```python
from build123d import *

# Parameters (mm, degrees)
F1_DEPTH       = 110
F0_W           = 30
F0_H           = 30
F2_DEPTH       = 3.36
F3_R           = 2
F5_D           = 8
F5_DEPTH       = 4
F7_D           = 4
F7_DEPTH       = 4
F7_CSINK_D     = 8
F7_CSINK_ANGLE = 90
F8_W           = 30
F8_H           = 13
F9_DEPTH       = 1


with BuildPart() as f1:
    # F0 (on Top) → F1 (new body)
    with BuildSketch(Plane.XY):
        Polygon((15, -18.36), (15, -15), (-15, -15), (-15, 15), (15, 15), (15, 18.36), (-18.36, 18.36), (-18.36, -18.36), align=None)
    extrude(amount=F1_DEPTH)

    # F0 (on Top) → F2 (join)
    with BuildSketch(Plane.XY):
        Rectangle(F0_W, F0_H)
    extrude(amount=F2_DEPTH)

    # F3
    f3_edges = [f1.edges().sort_by_distance(p)[0] for p in [
        (-18.36, -18.36, 55),
        (-18.36, 18.36, 55),
        (15, -18.36, 55),
        (15, 18.36, 55),
    ]]
    fillet(f3_edges, radius=F3_R)

    # F5
    with Locations(Plane.XZ.offset(18.36)):
        with Locations((0, 30), (0, 80)):
            Hole(F5_D / 2, depth=F5_DEPTH)

    # F7
    with Locations(Plane.XZ.offset(-15)):
        with Locations((0, 30), (0, 80)):
            CounterSinkHole(F7_D / 2, F7_CSINK_D / 2, depth=F7_DEPTH, counter_sink_angle=F7_CSINK_ANGLE)

    # F8 (on face) → F9 (cut)
    with BuildSketch(Plane(origin=(0, -15, 0), x_dir=(-1, 0, 0), z_dir=(0, 1, 0))):
        with Locations((0, 16.86)):
            Rectangle(F8_W, F8_H)
    extrude(amount=-F9_DEPTH, mode=Mode.SUBTRACT)


solid = f1.part
```
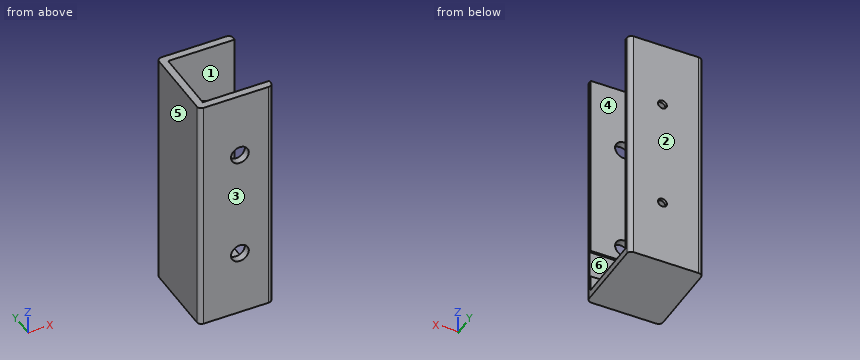
Read the model definition and answer for the solid it produces. Units are mm, in the model's axes. Face numbers are marked on the shaded views. A direction names the side the tool comes from. Coordinates: 2 decimals unless noted, no trailing zeros. Write each loop counter-clockwise with the first axis right and the second up, starting at its lowest first coordinate (ties: lowest second). Pieces come first, ordered by that corner, then holes. Notation, with made-up numbers: (85.25, -14) - (114.25, -14) arc R6 cw to (114.25, -10) - close; hole circle Ø11 at (-30.75, 79). An arc over 180 degrees is marked (long way). Answer as a JSON object with one key per item and string values. Group by question number.
1. The mould has two halves that part along Y. Classify the marked faces 1, 2 and 3: +Y half, -Y half, draft (parallel to the pull), parting line (faces both ways), or undercut.
2. A cutting plane is placed at D-D (z = 61.5). Determine the outline of the cut face in (x, y).
3. Each of these flat-tipped pins is pushed along its axis until it touches: P1, Ø8, axis at x = -2.5, y = -10.5, coming from the +Z side; P2, Ø4.5, axis at x = 0, z = 80, coming from the -Y side; P3, Ø12, axis at y = -7, z = 55.5, coming from the +X side. Where does it stop, or does it pass through?
4. A cutting plane is placed at C-C (y = -8). Determine the outline of the cut face in (x, z), plus the area to 3 significant figures.
5. Which of the six approach directions +Z, -Z, +X, -X, +Y, -Y give full straight-line access (tool end or side, diameter ignored) to the marked faces 4, 5 and 6?
6. A cutting plane is placed at B-B (x = 0). Give the number of separate pieces and of enclosed holes in the cut face, plus the area to 3 significant figures.
7. Consider L1, parallel to Z at x = 0, y = -16.95; L2, parallel to Y at x = -11, z = 34.5; L3, parallel to Z at x = 0, y = 17. Determine where each line is inside the solid, lowest interval first. Write a range as [from, to].
8. A cutting plane is placed at A-A (z = 30). Determine the outline of the cut face in (x, y), plus the area to 3 significant figures.
Worked out:
{
 "1": {"face 1": "undercut", "face 2": "+Y half", "face 3": "-Y half"},
 "2": {"outline": "(-18.36, -16.36) arc R2 ccw to (-16.36, -18.36) - (13, -18.36) arc R2 ccw to (15, -16.36) - (15, -15) - (-15, -15) - (-15, 15) - (15, 15) - (15, 16.36) arc R2 ccw to (13, 18.36) - (-16.36, 18.36) arc R2 ccw to (-18.36, 16.36) - close"},
 "3": {"P1": "stops at z = 3.36", "P2": "stops at y = 16.75", "P3": "stops at x = -15"},
 "4": {"outline": "(-18.36, 0) - (15, 0) - (15, 3.36) - (-15, 3.36) - (-15, 110) - (-18.36, 110) - close", "area": "470 mm²"},
 "5": {"face 4": "+Z, +X", "face 5": "+Z, -Z, -X, +Y, -Y", "face 6": "+X"},
 "6": {"separate pieces": "5", "enclosed holes": "0", "area": "738 mm²"},
 "7": {"L1": "z = [0, 26], [34, 76], [84, 110]", "L2": "y = [-18.36, -15], [15, 18.36]", "L3": "z = [0, 28], [32, 78], [82, 110]"},
 "8": {"outline": "(-18.36, -16.36) arc R2 ccw to (-16.36, -18.36) - (-4, -18.36) - (-4, -15) - (-15, -15) - (-15, 15) - (-4, 15) - (-2, 17) - (-2, 18.36) - (-16.36, 18.36) arc R2 ccw to (-18.36, 16.36) - close; (2, 17) - (4, 15) - (15, 15) - (15, 16.36) arc R2 ccw to (13, 18.36) - (2, 18.36) - close; (4, -18.36) - (13, -18.36) arc R2 ccw to (15, -16.36) - (15, -15) - (4, -15) - close", "area": "277 mm²"}
}
